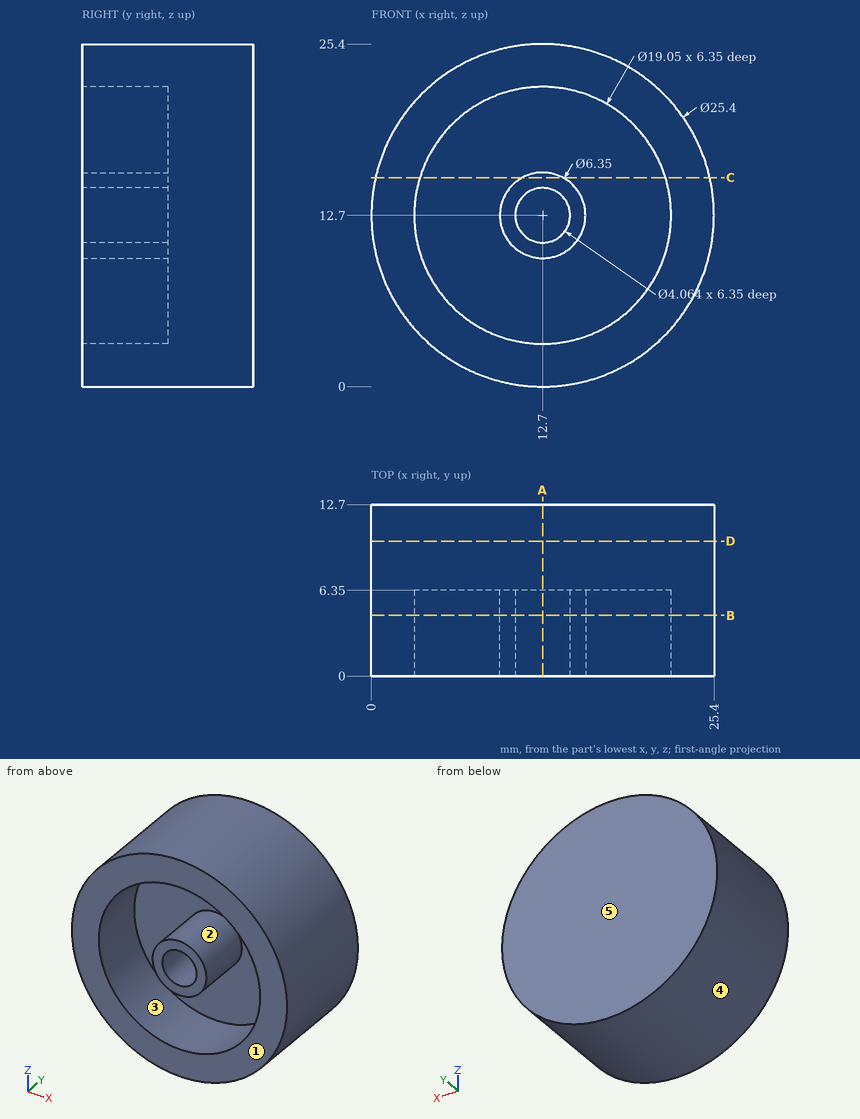
Could you check a few things on this drawing? It's one solid part, dimensions in mm from its lowest x, y, z. A direction names the side the tool comes from. Round coordinates to 2 decimals unless told otherwise and drop trailing zeros. Write each loop counter-clockwise with the first axis right and the second up, starting at its lowest first coordinate (ties: lowest second). Pieces come first, ordered by that corner, then holes. Notation, with made-up numbers: (44, 2) -> (82, 2) arc R15 ccw to (82, 22) -> close; hole circle Ø3 at (76, 88.5). An arc over 180 degrees is marked (long way). One line per question, with ' | ' between items. Start each with the question number.
1) Suppose I cut it at B-B on y = 4.5. Write out the boundary of the cut face in (x, z) (3 decimals).
2) Suppose I cut it at C-C on z = 15.5. Write out the boundary of the cut face in (x, y).
3) If we mould it in two halves opening along X, with no side actions, what happens to the marked faces 3, 4 and 5? For each: released by +X, released by -X, zero draft, split by the parting line, or undercut.
4) Suppose I cut it at A-A on x = 12.7. Write out the boundary of the cut face in (y, z) (3 decimals), then the cut area to 3 significant figures.
5) I need wall thicknesses on line 1 (Z direction, x = 12.7, y = 1.5) (3 decimals); line 2 (X direction, y = 4, z = 15.5); line 3 (Z direction, x = 11.5, y = 1). Which ranges of each line are inside material? Lowest first, please. Write a range as [from, to].
6) I'm going to push flat-ended pins straight in: P1, Ø2, axis at y = 3, z = 5.5, coming from the -X side; P2, Ø3, axis at x = 8, y = 6, coming from the -Z side; P3, Ø4, axis at y = 3, z = 19, coming from the -X side. Where does each tip first touch, or does it pass through?
7) Suppose I cut it at D-D on y = 10. Write out the boundary of the cut face in (x, z), then the cut area to 3 significant figures.
8) On a 3-axis mill with a long thin cutter (end or side, diameter ignored), from which of +Z, -Z, +X, -X, +Y, -Y can I reach the whole of each face in a straight line? I mean the marked faces 1 and 2. Say none if no direction works.
Return value:
1) outline: circle Ø25.4 at (12.7, 12.7); circle Ø6.35 at (12.7, 12.7); hole circle Ø19.05 at (12.7, 12.7); hole circle Ø4.064 at (12.7, 12.7)
2) outline: (0.31, 0) -> (3.6, 0) -> (3.6, 6.35) -> (11.2, 6.35) -> (11.2, 0) -> (14.2, 0) -> (14.2, 6.35) -> (21.8, 6.35) -> (21.8, 0) -> (25.09, 0) -> (25.09, 12.7) -> (0.31, 12.7) -> close
3) face 3: undercut | face 4: split by the parting line | face 5: zero draft
4) outline: (0, 0) -> (12.7, 0) -> (12.7, 25.4) -> (0, 25.4) -> (0, 22.225) -> (6.35, 22.225) -> (6.35, 15.875) -> (0, 15.875) -> (0, 14.732) -> (6.35, 14.732) -> (6.35, 10.668) -> (0, 10.668) -> (0, 9.525) -> (6.35, 9.525) -> (6.35, 3.175) -> (0, 3.175) -> close | area: 216 mm2
5) line 1: z = [0, 3.175], [9.525, 10.668], [14.732, 15.875], [22.225, 25.4] | line 2: x = [0.31, 3.6], [11.2, 14.2], [21.8, 25.09] | line 3: z = [0.06, 3.25], [9.76, 11.06], [14.34, 15.64], [22.15, 25.34]
6) P1: stops at x = 1.62 | P2: stops at z = 0.41 | P3: stops at x = 0.75
7) outline: circle Ø25.4 at (12.7, 12.7) | area: 507 mm2
8) face 1: +Z, -Z, +X, -X, -Y | face 2: -Y
